```python
from build123d import *

# Parameters (mm, degrees)
BOSS_EXTRUDE1_DEPTH = 2.25
BOSS_EXTRUDE2_DEPTH = 2.249999945
SKETCH4_W           = 3.683
SKETCH4_H           = 4.5
BOSS_EXTRUDE3_DEPTH = 1.143


with BuildPart() as part:
    # Sketch1 → Boss-Extrude1 (new body, symmetric)
    with BuildSketch(Plane.XY):
        with BuildLine():
            Line((0, 10.45), (0, -10.45))
            Line((0, -10.45), (3.175, -10.45))
            Line((3.175, -10.45), (3.175, -14.95))
            Line((3.175, -14.95), (8.255, -14.95))
            Line((8.255, -14.95), (8.255, -10.45))
            Line((8.255, -10.45), (11.43, -10.45))
            Line((11.43, -10.45), (11.43, 9.125))
            ThreePointArc((11.43, 9.125), (12.35993597, 11.37006403), (14.605, 12.3))
            Line((14.605, 12.3), (15.875, 12.3))
            Line((15.875, 12.3), (15.875, 15.475))
            Line((15.875, 15.475), (9.525, 15.475))
            Line((9.525, 15.475), (9.525, 19.975))
            Line((9.525, 19.975), (15.875, 19.975))
            Line((15.875, 19.975), (15.875, 23.15))
            Line((15.875, 23.15), (3.683, 23.15))
            Line((3.683, 23.15), (3.683, 10.45))
            Line((3.683, 10.45), (0, 10.45))
        make_face()
    extrude(amount=BOSS_EXTRUDE1_DEPTH, both=True)

    # Sketch2 → Boss-Extrude2 (add, symmetric)
    with BuildSketch(Plane.XY):
        Polygon((3.683, 23.15), (4.953, 26.325), (10.375738686, 26.325), (15.875, 23.15), align=None)
    extrude(amount=BOSS_EXTRUDE2_DEPTH, both=True)

    # Sketch4 → Boss-Extrude3 (add)
    with BuildSketch(Plane(origin=(0, 8.545, 0), x_dir=(1, 0, 0), z_dir=(0, 1, 0))):
        with Locations((1.8415, 0)):
            Rectangle(SKETCH4_W, SKETCH4_H)
    extrude(amount=BOSS_EXTRUDE3_DEPTH)


solid = part.part
```
Work out the finished part from the listing and answer in its coordinate system (mm). A direction names the side the tool comes from. Round coordinates to 2 decimals unless told otherwise and drop trailing zeros. Loops run counter-clockwise (first coordinate to the right, second up) from the corner with the lowest first, then second, coordinate; pieces in that order, holes last.
(1) Each of these flat-tipped pins is pushed along its axis until it touches: P1, Ø1.6, axis at x = 10, z = -1, coming from the -Y side; P2, Ø1.4, axis at x = 15, z = 0, coming from the -Y side; P3, Ø2, axis at y = 18, z = -1, coming from the +X side (3 decimals). Where does it stop, or does it pass through?
Computed values:
P1: stops at y = -10.45
P2: stops at y = 12.29
P3: stops at x = 9.525
(2) The part is cut by section C-C, the plane y = 13. Give the vertices of the cut face in (x, z) (3 decimals), and give its area (3 significant figures).
Computed values:
outline: (3.683, -2.25) - (15.875, -2.25) - (15.875, 2.25) - (3.683, 2.25) - close
area: 54.9 mm2
(3) The part is cut by section D-D, the plane x = 2.25. Give the vertices of the cut face in (y, z).
Computed values:
outline: (-10.45, -2.25) - (10.45, -2.25) - (10.45, 2.25) - (-10.45, 2.25) - close
(4) Find the intervals of material crossed by L1, parallel to X at y = 1, z = 0.3; L2, parallel to Y at x = 10.75, z = 1.7 (3 decimals); L3, parallel to Y at x = 12, z = -0.7 (3 decimals), in increasing order.
Computed values:
L1: x = 0 to 11.43
L2: y = -10.45 to 15.475, 19.975 to 26.109
L3: y = 10.94 to 15.475, 19.975 to 25.387
(5) The part is cut by section A-A, the plane z = 0.75. Give the vertices of the cut face in (x, y) (3 decimals), and give its area (3 significant figures).
Computed values:
outline: (0, -10.45) - (3.175, -10.45) - (3.175, -14.95) - (8.255, -14.95) - (8.255, -10.45) - (11.43, -10.45) - (11.43, 9.125) arc R3.175 cw to (14.605, 12.3) - (15.875, 12.3) - (15.875, 15.475) - (9.525, 15.475) - (9.525, 19.975) - (15.875, 19.975) - (15.875, 23.15) - (10.376, 26.325) - (4.953, 26.325) - (3.683, 23.15) - (3.683, 10.45) - (0, 10.45) - close
area: 410 mm2
(6) The part is cut by section B-B, the plane x = 11. Give the vertices of the cut face in (y, z) (3 decimals), and give its area (3 significant figures).
Computed values:
outline: (-10.45, -2.25) - (15.475, -2.25) - (15.475, 2.25) - (-10.45, 2.25) - close; (19.975, -2.25) - (25.965, -2.25) - (25.965, 2.25) - (19.975, 2.25) - close
area: 144 mm2
(7) For faces 4 (the flat face through (2, -10.45, 0)), 5 (the flat face through (13, 15.475, 0)), 6 (the flat face through (6, 6, -2.25)), 7 (the flat face through (15, 12.3, 0)), 8 (the flat face through (2, 10.45, 0)), determine the directions among +Z, -Z, +X, -X, +Y, -Y from which every point of the face is accessible in a straight line to the end or side of a thin tool.
Computed values:
face 4: +Z, -Z, -X, -Y
face 5: +Z, -Z, +X
face 6: -Z, +X, -X, +Y, -Y
face 7: +Z, -Z, +X, -Y
face 8: +Z, -Z, -X, +Y
(8) The mould has two halves that part along Y. Classify faces 1 (the flat face through (13, 19.975, 0)), 2 (the flat face through (3.175, -13, 0)), 3 (the flat face through (13.09, 24.76, 0.03)): pulls with the +Y half, pulls with the -Y half, needs draft (parallel to the pull), parting line crosses it, or undercut.
Computed values:
face 1: undercut
face 2: needs draft
face 3: pulls with the +Y half
